Read the model definition and answer for the solid it produces. Units are mm, in the model's axes. Face numbers are marked on the shaded views. A direction names the side the tool comes from. Coordinates: 2 decimals unless noted, no trailing zeros. Order: outer loops, then holes, each group sorted by start corner. A loop starts at its lowest first (then second) coordinate and runs counter-clockwise, first axis right, second up. Notation, with made-up numbers: M -35.75,87 L -13.75,87 A28 cw -13.75,117 Z; hole C 85,24 d8. An arc over 180 degrees is marked long. Put each result on its own line as item: value.
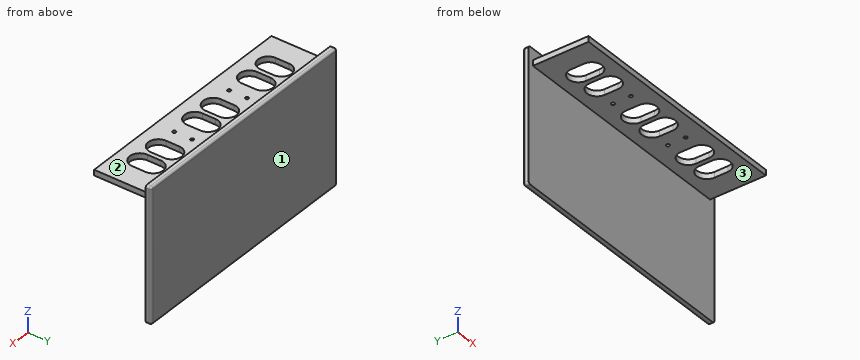
from build123d import *

# Parameters (mm, degrees)
CROQUIS1_W              = 220
CROQUIS1_H              = 120
SALIENTE_EXTRUIR1_DEPTH = 5
CROQUIS2_W              = 210
CROQUIS2_H              = 5
SALIENTE_EXTRUIR2_DEPTH = 50
CORTAR_EXTRUIR1_REACH   = 165.401
REDONDEO1_R             = 2
CORTAR_EXTRUIR3_REACH   = 165.401
CROQUIS11_R             = 1.5


with BuildPart() as part:
    # Croquis1 → Saliente-Extruir1 (new body)
    with BuildSketch(Plane(origin=(0, 0, 0), x_dir=(1, 0, 0), z_dir=(0, 1, 0))):
        Rectangle(CROQUIS1_W, CROQUIS1_H)
    extrude(amount=SALIENTE_EXTRUIR1_DEPTH)

    # Croquis2 → Saliente-Extruir2 (add)
    with BuildSketch(Plane.XZ):
        with Locations((0, 47.5)):
            Rectangle(CROQUIS2_W, CROQUIS2_H)
    extrude(amount=SALIENTE_EXTRUIR2_DEPTH)

    # Croquis3 → Cortar-Extruir1 (cut, up to next)
    with BuildSketch(Plane.XY.offset(50), mode=Mode.PRIVATE) as cortar_extruir1_sk1:
        with BuildLine():
            Line((-45, -19), (-45, -31))
            ThreePointArc((-45, -31), (-54, -40), (-63, -31))
            Line((-63, -31), (-63, -19))
            ThreePointArc((-63, -19), (-54, -10), (-45, -19))
        make_face()
    cortar_extruir1_tool1 = extrude(cortar_extruir1_sk1.sketch, amount=-CORTAR_EXTRUIR1_REACH, mode=Mode.PRIVATE) & part.part
    # Croquis3 → Cortar-Extruir1 (cut, up to next)
    with BuildSketch(Plane.XY.offset(50), mode=Mode.PRIVATE) as cortar_extruir1_sk2:
        with BuildLine():
            Line((-85, -19), (-85, -31))
            ThreePointArc((-85, -31), (-76, -40), (-67, -31))
            Line((-67, -31), (-67, -19))
            ThreePointArc((-67, -19), (-76, -10), (-85, -19))
        make_face()
    cortar_extruir1_tool2 = extrude(cortar_extruir1_sk2.sketch, amount=-CORTAR_EXTRUIR1_REACH, mode=Mode.PRIVATE) & part.part
    # Croquis3 → Cortar-Extruir1 (cut, up to next)
    with BuildSketch(Plane.XY.offset(50), mode=Mode.PRIVATE) as cortar_extruir1_sk3:
        with BuildLine():
            Line((20, -19), (20, -31))
            ThreePointArc((20, -31), (11, -40), (2, -31))
            Line((2, -31), (2, -19))
            ThreePointArc((2, -19), (11, -10), (20, -19))
        make_face()
    cortar_extruir1_tool3 = extrude(cortar_extruir1_sk3.sketch, amount=-CORTAR_EXTRUIR1_REACH, mode=Mode.PRIVATE) & part.part
    # Croquis3 → Cortar-Extruir1 (cut, up to next)
    with BuildSketch(Plane.XY.offset(50), mode=Mode.PRIVATE) as cortar_extruir1_sk4:
        with BuildLine():
            Line((-2, -19), (-2, -31))
            ThreePointArc((-2, -31), (-11, -40), (-20, -31))
            Line((-20, -31), (-20, -19))
            ThreePointArc((-20, -19), (-11, -10), (-2, -19))
        make_face()
    cortar_extruir1_tool4 = extrude(cortar_extruir1_sk4.sketch, amount=-CORTAR_EXTRUIR1_REACH, mode=Mode.PRIVATE) & part.part
    # Croquis3 → Cortar-Extruir1 (cut, up to next)
    with BuildSketch(Plane.XY.offset(50), mode=Mode.PRIVATE) as cortar_extruir1_sk5:
        with BuildLine():
            Line((85, -19), (85, -31))
            ThreePointArc((85, -31), (76, -40), (67, -31))
            Line((67, -31), (67, -19))
            ThreePointArc((67, -19), (76, -10), (85, -19))
        make_face()
    cortar_extruir1_tool5 = extrude(cortar_extruir1_sk5.sketch, amount=-CORTAR_EXTRUIR1_REACH, mode=Mode.PRIVATE) & part.part
    # Croquis3 → Cortar-Extruir1 (cut, up to next)
    with BuildSketch(Plane.XY.offset(50), mode=Mode.PRIVATE) as cortar_extruir1_sk6:
        with BuildLine():
            Line((63, -19), (63, -31))
            ThreePointArc((63, -31), (54, -40), (45, -31))
            Line((45, -31), (45, -19))
            ThreePointArc((45, -19), (54, -10), (63, -19))
        make_face()
    cortar_extruir1_tool6 = extrude(cortar_extruir1_sk6.sketch, amount=-CORTAR_EXTRUIR1_REACH, mode=Mode.PRIVATE) & part.part
    add(cortar_extruir1_tool1.solids().sort_by_distance((-54, -25, 50))[0], mode=Mode.SUBTRACT)
    add(cortar_extruir1_tool2.solids().sort_by_distance((-76, -25, 50))[0], mode=Mode.SUBTRACT)
    add(cortar_extruir1_tool3.solids().sort_by_distance((11, -25, 50))[0], mode=Mode.SUBTRACT)
    add(cortar_extruir1_tool4.solids().sort_by_distance((-11, -25, 50))[0], mode=Mode.SUBTRACT)
    add(cortar_extruir1_tool5.solids().sort_by_distance((76, -25, 50))[0], mode=Mode.SUBTRACT)
    add(cortar_extruir1_tool6.solids().sort_by_distance((54, -25, 50))[0], mode=Mode.SUBTRACT)

    # Redondeo1
    redondeo1_edges = [part.edges().sort_by_distance(p)[0] for p in [
        (-110, 5, 0),
        (0, 5, 60),
        (110, 5, 0),
        (110, 2.5, 60),
        (-110, 2.5, 60),
        (-110, 2.5, -60),
        (110, 2.5, -60),
        (0, 5, -60),
    ]]
    fillet(redondeo1_edges, radius=REDONDEO1_R)

    # Croquis11 → Cortar-Extruir3 (cut, up to next)
    with BuildSketch(Plane.XY.offset(50), mode=Mode.PRIVATE) as cortar_extruir3_sk1:
        with Locations((-32.5, -17)):
            Circle(CROQUIS11_R)
    cortar_extruir3_tool1 = extrude(cortar_extruir3_sk1.sketch, amount=-CORTAR_EXTRUIR3_REACH, mode=Mode.PRIVATE) & part.part
    # Croquis11 → Cortar-Extruir3 (cut, up to next)
    with BuildSketch(Plane.XY.offset(50), mode=Mode.PRIVATE) as cortar_extruir3_sk2:
        with Locations((-32.5, -33)):
            Circle(CROQUIS11_R)
    cortar_extruir3_tool2 = extrude(cortar_extruir3_sk2.sketch, amount=-CORTAR_EXTRUIR3_REACH, mode=Mode.PRIVATE) & part.part
    # Croquis11 → Cortar-Extruir3 (cut, up to next)
    with BuildSketch(Plane.XY.offset(50), mode=Mode.PRIVATE) as cortar_extruir3_sk3:
        with Locations((32.5, -17)):
            Circle(CROQUIS11_R)
    cortar_extruir3_tool3 = extrude(cortar_extruir3_sk3.sketch, amount=-CORTAR_EXTRUIR3_REACH, mode=Mode.PRIVATE) & part.part
    # Croquis11 → Cortar-Extruir3 (cut, up to next)
    with BuildSketch(Plane.XY.offset(50), mode=Mode.PRIVATE) as cortar_extruir3_sk4:
        with Locations((32.5, -33)):
            Circle(CROQUIS11_R)
    cortar_extruir3_tool4 = extrude(cortar_extruir3_sk4.sketch, amount=-CORTAR_EXTRUIR3_REACH, mode=Mode.PRIVATE) & part.part
    add(cortar_extruir3_tool1.solids().sort_by_distance((-32.5, -17, 50))[0], mode=Mode.SUBTRACT)
    add(cortar_extruir3_tool2.solids().sort_by_distance((-32.5, -33, 50))[0], mode=Mode.SUBTRACT)
    add(cortar_extruir3_tool3.solids().sort_by_distance((32.5, -17, 50))[0], mode=Mode.SUBTRACT)
    add(cortar_extruir3_tool4.solids().sort_by_distance((32.5, -33, 50))[0], mode=Mode.SUBTRACT)


solid = part.part
Q1. Find section A-A on y = -23.5. Write down the section's boundary in (x, z), plus the area to 3 significant figures.
Answers below:
outline: M -105,45 L -85,45 L -85,50 L -105,50 Z; M -67,45 L -63,45 L -63,50 L -67,50 Z; M -45,45 L -20,45 L -20,50 L -45,50 Z; M -2,45 L 2,45 L 2,50 L -2,50 Z; M 20,45 L 45,45 L 45,50 L 20,50 Z; M 63,45 L 67,45 L 67,50 L 63,50 Z; M 85,45 L 105,45 L 105,50 L 85,50 Z
area: 510 mm^2
Q2. Find section D-D on y = -45. Write down the section's boundary in (x, z).
Answers below:
outline: M -105,45 L 105,45 L 105,50 L -105,50 Z
Q3. Given pin 1 (6 mm diameter, centred on x = 22.5, y = -18.5, fed in from +Z); pin 2 (4 mm diameter, centred on y = -24.5, z = 47, fed in from +X); pin 3 (2.5 mm diameter, centred on x = 32.5, y = -33, fed in from +Z); pin 4 (1.5 mm diameter, centred on y = -26.5, z = 46.5, fed in from -X), each flat-ended and moving along its own axis, determine where each tip first touches the part or whether it passes through.
Answers below:
pin 1: stops at z = 50
pin 2: stops at x = 105
pin 3: passes through
pin 4: stops at x = -105
Q4. Consider line 1 along Y through (x, z) = (32.5, 47.1); line 2 along Y through (x, z) = (70, -2.5); line 3 along Z through (x, y) = (-42.5, -25). Determine where each line is inside the solid, lowest interval first.
Answers below:
line 1: y = -50 to -34.5, -31.5 to -18.5, -15.5 to 5
line 2: y = 0 to 5
line 3: z = 45 to 50
Q5. A tool of negligible diameter and unlimited length cuts with its end or side. For the marked faces 1, 2 and 3, from which of +Z, -Z, +X, -X, +Y, -Y can it reach the whole face along a straight path? Write none if from no direction.
Answers below:
face 1: +Z, -Z, +X, -X, +Y
face 2: +Z, +X, -X, -Y
face 3: -Z, +X, -X, -Y
Q6. Find section B-B on x = 54. Write down the section's boundary in (y, z), plus the area to 3 significant figures.
Answers below:
outline: M -50,45 L -40,45 L -40,50 L -50,50 Z; M -10,45 L 0,45 L 0,-60 L 3,-60 A2 ccw 5,-58 L 5,58 A2 ccw 3,60 L 0,60 L 0,50 L -10,50 Z
area: 698 mm^2
Q7. Find section C-C on z = -28. Write down the section's boundary in (x, y), plus the area to 3 significant figures.
Answers below:
outline: M -110,0 L 110,0 L 110,3 A2 ccw 108,5 L -108,5 A2 ccw -110,3 Z
area: 1,100 mm^2
